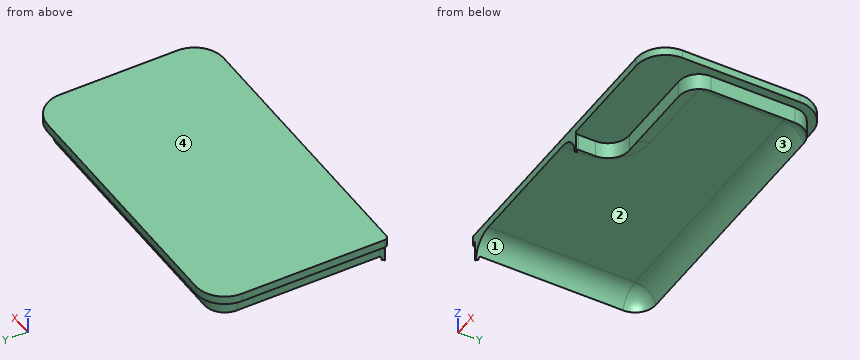
```python
from build123d import *

# Parameters (mm, degrees)
SKETCH1_W           = 74
SKETCH1_H           = 42
BOSS_EXTRUDE1_DEPTH = 2
BOSS_EXTRUDE2_DEPTH = 5
FILLET2_R           = 5
FILLET3_R           = 5
FILLET4_R           = 7
CUT_EXTRUDE2_DEPTH  = 5
FILLET6_R           = 1


with BuildPart() as part:
    # Sketch1 → Boss-Extrude1 (new body)
    with BuildSketch(Plane.XY):
        Rectangle(SKETCH1_W, SKETCH1_H)
    extrude(amount=BOSS_EXTRUDE1_DEPTH)

    # Sketch2 → Boss-Extrude2 (add)
    with BuildSketch(Plane(origin=(0, 0, 0), x_dir=(-1, 0, 0), z_dir=(0, 0, -1))):
        Polygon((37, 21), (-37, 21), (-37, -21), (-5, -21), (-5, -11), (-35, -11), (-35, 19), (35, 19), (35, -21), (37, -21), align=None)
    extrude(amount=BOSS_EXTRUDE2_DEPTH)

    # Fillet2
    fillet2_edges = [part.edges().sort_by_distance(p)[0] for p in [
        (5, -11, -2.5),
        (35, -11, -2.5),
        (35, 19, -2.5),
        (-35, 19, -2.5),
    ]]
    fillet(fillet2_edges, radius=FILLET2_R)

    # Fillet3
    fillet3_edges = [part.edges().sort_by_distance(p)[0] for p in [
        (5, -18.5, 0),
        (6.464466094, -12.464466094, 0),
        (20, -11, 0),
        (33.535533906, -9.535533906, 0),
        (35, 4, 0),
        (33.535533906, 17.535533906, 0),
        (-35, -3.5, 0),
        (-33.535533906, 17.535533906, 0),
        (0, 19, 0),
    ]]
    fillet(fillet3_edges, radius=FILLET3_R - 0.0001)  # a hair under: the kernel refuses the full size

    # Fillet4
    fillet4_edges = [part.edges().sort_by_distance(p)[0] for p in [
        (-37, 21, -1.5),
        (37, 21, -1.5),
        (37, -21, -1.5),
    ]]
    fillet(fillet4_edges, radius=FILLET4_R)

    # Sketch3 → Cut-Extrude2 (cut)
    with BuildSketch(Plane(origin=(0, 0, 0), x_dir=(-1, 0, 0), z_dir=(0, 0, -1))):
        with BuildLine():
            Line((37.1, 21.1), (-37.1, 21.1))
            Line((-37.1, 21.1), (-37.1, -21.1))
            Line((-37.1, -21.1), (-6, -21.1))
            ThreePointArc((-6, -21.1), (-5.222182541, -20.777817459), (-4.9, -20))
            Line((-4.9, -20), (-4.9, -16))
            ThreePointArc((-4.9, -16), (-6.393755416, -12.393755416), (-10, -10.9))
            Line((-10, -10.9), (-30, -10.9))
            ThreePointArc((-30, -10.9), (-33.464823228, -9.464823228), (-34.9, -6))
            Line((-34.9, -6), (-34.9, 14))
            ThreePointArc((-34.9, 14), (-33.464823228, 17.464823228), (-30, 18.9))
            Line((-30, 18.9), (30, 18.9))
            ThreePointArc((30, 18.9), (33.464823228, 17.464823228), (34.9, 14))
            Line((34.9, 14), (34.9, -20))
            ThreePointArc((34.9, -20), (35.222182541, -20.777817459), (36, -21.1))
            Line((36, -21.1), (37.1, -21.1))
            Line((37.1, -21.1), (37.1, 21.1))
        make_face()
    extrude(amount=CUT_EXTRUDE2_DEPTH, mode=Mode.SUBTRACT)

    # Fillet6
    fillet6_edges = [part.edges().sort_by_distance(p)[0] for p in [
        (-37, -21, 1),
    ]]
    fillet(fillet6_edges, radius=FILLET6_R)


solid = part.part
```
Can you work these out from the model? Positions are in its coordinate system, mm. Face numbers are marked on the shaded views. A direction names the side the tool comes from. Give positions to 0.01 mm unless a question says otherwise; leave off trailing zeros. Loops run counter-clockwise (first coordinate to the right, second up) from the corner with the lowest first, then second, coordinate; pieces in that order, holes last. Notation, with made-up numbers: M 25.5,21 L 64.5,21 A24 cw 64.5,42 Z; hole C 8.25,83.25 d10. An arc over 180 degrees is marked long. Use one line per item in the form item = value. Start each with the question number.
(1) Thinking about a two-plate mould opening in Y: for the marked faces 3 and 4, which applies, released by +Y, released by -Y, zero draft, split by the parting line, or undercut?
(2) I'm going to push flat-ended pins straight in: P1, Ø21, axis at x = -6.5, y = -6, coming from the -Z side; P2, Ø6, axis at x = 3, y = 5, coming from the -Z side; P3, Ø2, axis at y = -10.5, z = -3, coming from the -X side. Where does each tip first touch, or does it pass through?
(3) I want a section at C-C, the plane x = -14.5. Write out the boundary of the cut face in (y, z), and give its area (3 significant figures).
(4) I want a section at B-B, the plane y = 11. Write out the boundary of the cut face in (x, z).
(5) On a 3-axis mill with a long thin cutter (end or side, diameter ignored), from which of +Z, -Z, +X, -X, +Y, -Y can I reach the whole of each face in a straight line? I mean the marked faces 1 and 2. Say none if no direction works.
(6) I want a section at A-A, the plane x = 26.5. Write out the boundary of the cut face in (y, z).
(7) Please list where these lines run through material, in increasing order: line 1 (Z direction, x = 6, y = 12); line 2 (X direction, y = -5, z = -0.75); line 3 (X direction, y = 2.5, z = -0.5).
Worked out:
q1.face_3 = undercut
q1.face_4 = zero draft
q2.P1 = -0.15
q2.P2 = 0
q2.P3 = -34.9
q3.outline = M -21,0 L 14,0 A5 cw 18.9,-4 L 18.9,0 L 21,0 L 21,2 L -21,2 Z
q3.area = 88.9 mm²
q4.outline = M -37,0 L -34.9,0 L -34.9,-4 A5 cw -30,0 L 30,0 A5 cw 34.9,-4 L 34.9,0 L 37,0 L 37,2 L -37,2 Z
q5.face_1 = -Z, -Y
q5.face_2 = -Z
q6.outline = M -21,0 L -10.9,0 L -10.9,-4 A5 cw -6,0 L 14,0 A5 cw 18.9,-4 L 18.9,0 L 21,0 L 21,2 L -21,2 Z
q7.line_1 = 0 to 2
q7.line_2 = -34.9 to -32.63, 32.63 to 34.9
q7.line_3 = -34.9 to -32.18, 32.18 to 34.9
